Can you work these out from the model? Positions are in its coordinate system, mm. A direction names the side the tool comes from. Give positions to 0.01 mm unless a question says otherwise; leave off trailing zeros. Order: outer loops, then holes, each group sorted by start corner. A loop starts at its lowest first (then second) coordinate and runs counter-clockwise, first axis right, second up. Notation, with made-up numbers: M 7.5,85 L 11.5,85 A28 cw 11.5,110 Z; hole C -33,63.5 d7. An arc over 180 degrees is marked long. Use a Markdown table: item, result. Add a question column.
Autodesk Inventor part; units mm, degrees
ref_plane "YZ Plane" through (0, 0, 0) normal (1, 0, 0) x (0, 1, 0)
ref_plane "XZ Plane" through (0, 0, 0) normal (0, 1, 0) x (-1, 0, 0)
ref_plane "XY Plane" through (0, 0, 0) normal (0, 0, 1) x (1, 0, 0)
sketch "Sketch1" plane through (0, 0, 0) normal (0, 0, 1) x (1, 0, 0)
  line L0 (-75, -53) -> (75, -53)
  line L1 (75, -53) -> (75, 53)
  line L2 (75, 53) -> (-75, 53)
  line L3 (-75, 53) -> (-75, -53)
  line L4 (-75, -53) -> (75, 53) construction
  line L5 (75, -53) -> (-75, 53) construction
  line L6 (-72, 50) -> (72, 50)
  line L7 (72, 50) -> (72, -50)
  line L8 (72, -50) -> (-72, -50)
  line L9 (-72, -50) -> (-72, 50)
  line L10 (69, 47) -> (-69, 47)
  line L11 (-69, 47) -> (-69, -47)
  line L12 (-69, -47) -> (69, -47)
  line L13 (69, -47) -> (69, 47)
  point P0 (0, 0)
  dimension "d0" = 150
  dimension "d1" = 106
  dimension "d4" = 3
  dimension "d5" = 3
extrude "Extrusion1" add sketch "Sketch1" along normal blind 3 contours L3 L2 L1 L0 | L6 L7 L8 L9 | L13 L12 L11 L10
extrude "Extrusion2" add sketch "Sketch1" against normal blind 8 contours L6 L7 L8 L9
fillet "Fillet1" radius 2 8 edges at (-75, 53, 1.5) (-69, 47, -4) (-75, -53, 1.5) (-69, -47, -4) (69, -47, -4) (75, -53, 1.5) (69, 47, -4) (75, 53, 1.5)
chamfer "Chamfer1" distance 1 angle 45 4 edges at (-72, -50, -4) (72, -50, -4) (72, 50, -4) (-72, 50, -4)
chamfer "Chamfer2" distance 0.5 distance2 5 8 edges at (72, 0, -8) (0, -50, -8) (-72, 0, -8) (0, 50, -8) (71.5, -49.5, -8) (-71.5, -49.5, -8) (-71.5, 49.5, -8) (71.5, 49.5, -8) measured on face at (22.3333, 49, -8)
properties part number "ImageToStl.com_82d01a97-71ed-4804-91bd-9032aadffd37"
1. I need wall thicknesses on L1, parallel to Y at x = 42, z = -0.25; L2, parallel to X at y = 43.5, z = -3; L3, parallel to Z at x = -35.5, y = -12.5. Which ranges of each line are inside material? Lowest first, please. Write a range as [from, to].
2. Will these pins go through, and if not, where does the flat tip stop? pin 1 (1.5 mm diameter, centred on y = -13, z = -2, fed in from -X); pin 2 (1.5 mm diameter, centred on y = -23.5, z = -1.5, fed in from +X); pin 3 (3.5 mm diameter, centred on x = 28.5, z = -1.5, fed in from -Y); pin 4 (2.5 mm diameter, centred on y = -19.5, z = -5.5, fed in from -X) (3 decimals).
3. If we section it at A-A, the plane y = -36: List the corners of the cut face in (x, z) for me.
4. If we section it at B-B, the plane z = -1.5: List the corners of the cut face in (x, y) for me.
5. On a 3-axis mill with a long thin cutter (end or side, diameter ignored), from which of +Z, -Z, +X, -X, +Y, -Y can I reach the whole of each face in a straight line? I mean faces 5 (the face through (-69, 1, -4)), 6 (the face through (1, -50, -1)), 7 (the face through (-72, -1, -1)), 8 (the face through (-1, 50, -1)). Say none if no direction works.
6. We'd pull the mould along Y, two halves only. Please class faces 1 (the face through (-1, 1, 0)), 2 (the face through (-1, -47, -4)), 3 (the face through (0.994, 49.753, -5.465)), 4 (the face through (-1, 1, 3)): +Y half, -Y half, draft (parallel to the pull), parting line (faces both ways), or undercut.
7. If we section it at C-C, the plane x = 44.5: List the corners of the cut face in (y, z) for me.
Geometry results:
| question | item | result |
|---|---|---|
| 1 | L1 | y = [-50, -47], [47, 50] |
| 1 | L2 | x = [-72, -69], [69, 72] |
| 1 | L3 | z = [0, 3] |
| 2 | pin 1 | stops at x = -72 |
| 2 | pin 2 | stops at x = 72 |
| 2 | pin 3 | stops at y = -53 |
| 2 | pin 4 | stops at x = -71.875 |
| 3 | outline | M -75,0 L -72,0 L -72,-3 L -71.5,-8 L -69,-8 L -69,0 L 69,0 L 69,-8 L 71.5,-8 L 72,-3 L 72,0 L 75,0 L 75,3 L -75,3 Z |
| 4 | outline | M -72,-49 L -71,-50 L 71,-50 L 72,-49 L 72,49 L 71,50 L -71,50 L -72,49 Z; hole M -69,-45 A2 ccw -67,-47 L 67,-47 A2 ccw 69,-45 L 69,45 A2 ccw 67,47 L -67,47 A2 ccw -69,45 Z |
| 5 | face 5 | -Z |
| 5 | face 6 | -Z, +X, -X, -Y |
| 5 | face 7 | -Z, -X, +Y, -Y |
| 5 | face 8 | -Z, +X, -X, +Y |
| 6 | face 1 | undercut |
| 6 | face 2 | undercut |
| 6 | face 3 | +Y half |
| 6 | face 4 | draft |
| 7 | outline | M -53,0 L -50,0 L -50,-3 L -49.5,-8 L -47,-8 L -47,0 L 47,0 L 47,-8 L 49.5,-8 L 50,-3 L 50,0 L 53,0 L 53,3 L -53,3 Z |
